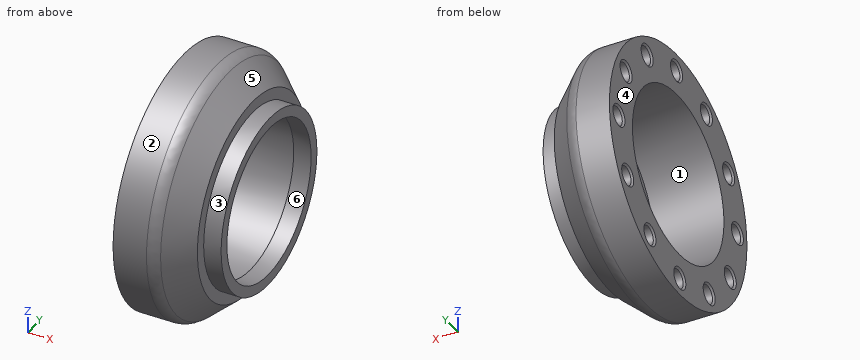
```python
from build123d import *

# Parameters (mm, degrees)
FILLET1_R                    = 10
SKETCH2_R                    = 50.53
SKETCH2_R_2                  = 44.45
BOSS_EXTRUDE1_DEPTH          = 10
SKETCH3_R                    = 5.35
CUT_EXTRUDE1_DEPTH           = 19.4
CHAMFER1_SIZE                = 1
CIRPATTERN1_COUNT            = 12
CHAMFER1_OF_CIRPATTERN1_SIZE = 1


with BuildPart() as part:
    # Sketch1 → Revolve1 (revolve)
    with BuildSketch(Plane.XY):
        Polygon((0, 48.25), (40, 48.25), (40, 57.15), (23, 72.5), (0, 72.5), align=None)
    revolve(axis=Axis((0, 0, 0), (1, 0, 0)))

    # Fillet1
    fillet1_edges = [part.edges().sort_by_distance(p)[0] for p in [
        (23, -72.5, 0),
    ]]
    fillet(fillet1_edges, radius=FILLET1_R)

    # Sketch2 → Boss-Extrude1 (add)
    with BuildSketch(Plane(origin=(40, 0, 0), x_dir=(0, 0, -1), z_dir=(1, 0, 0))):
        Circle(SKETCH2_R)
        Circle(SKETCH2_R_2, mode=Mode.SUBTRACT)
    extrude(amount=BOSS_EXTRUDE1_DEPTH)

    # Sketch3 → Cut-Extrude1 (cut)
    with BuildSketch(Plane.ZY):
        with Locations((-1.718407093, 62.47637215)):
            Circle(SKETCH3_R)
    cut_extrude1 = extrude(amount=-CUT_EXTRUDE1_DEPTH, mode=Mode.SUBTRACT)

    # Chamfer1
    chamfer1_edges = [part.edges().sort_by_distance(p)[0] for p in [
        (0, 62.47637215, -7.068407093),
    ]]
    chamfer(chamfer1_edges, length=CHAMFER1_SIZE)

    # CirPattern1: Cut-Extrude1 ×12 about axis
    cirpattern1_axis = Axis((0, 0, 0), (1, 0, 0))
    for i in range(1, CIRPATTERN1_COUNT):
        add(cut_extrude1.rotate(cirpattern1_axis, i * 360 / CIRPATTERN1_COUNT), mode=Mode.SUBTRACT)

    # Chamfer1 of CirPattern1
    chamfer1_of_cirpattern1_edges = [part.edges().sort_by_distance(p)[0] for p in [
        (0, 57.640328965, 25.116765969),
        (0, 37.359606182, 50.571921872),
        (0, 7.068407093, 62.47637215),
        (0, -25.116765969, 57.640328965),
        (0, -50.571921872, 37.359606182),
        (0, -62.47637215, 7.068407093),
        (0, -57.640328965, -25.116765969),
        (0, -37.359606182, -50.571921872),
        (0, -7.068407093, -62.47637215),
        (0, 25.116765969, -57.640328965),
        (0, 50.571921872, -37.359606182),
    ]]
    chamfer(chamfer1_of_cirpattern1_edges, length=CHAMFER1_OF_CIRPATTERN1_SIZE)


solid = part.part
```
The model under review builds one solid part; all positions refer to its coordinate system, in mm. Face numbers are marked on the shaded views. A direction names the side the tool comes from. Coordinates: 2 decimals unless noted, no trailing zeros. Loops run counter-clockwise (first coordinate to the right, second up) from the corner with the lowest first, then second, coordinate; pieces in that order, holes last. Notation, with made-up numbers: (74, 76.25) -> (80, 76.25) arc R17 cw to (80, 100.25) -> close; hole circle Ø6 at (71.5, 45.5). An arc over 180 degrees is marked (long way). Answer as CSV lines item,"result".
Item 1: Take a section at A-A, the plane x = 4. Count the separate pieces of the cut face and the enclosed holes in it, and give its area (3 significant figures).
Results below:
separate pieces,"1"
enclosed holes,"13"
area,"8,120 mm2"
Item 2: Insertion check: pin 1 (3 mm diameter, centred on y = -54.5, z = 33.5, fed in from -X); pin 2 (12 mm diameter, centred on y = 54, z = 23, fed in from +X); pin 3 (9.5 mm diameter, centred on y = 1.72, z = 62.48, fed in from +X). Each pin has a flat end and moves straight along its axis. Give the tip position at first contact, or say it passes through.
Results below:
pin 1,"stops at x = 19.4"
pin 2,"stops at x = 40"
pin 3,"stops at x = 39.33"
Item 3: Take a section at C-C, the plane x = 36. State the section outline as (y, z) points, and give its area (3 significant figures).
Results below:
outline,"circle Ø121.52 at (0, 0); hole circle Ø96.5 at (0, 0)"
area,"4,280 mm2"
Item 4: Machinability: for the marked faces 1, 2 and 3, which of the approach directions +Z, -Z, +X, -X, +Y, -Y give a long, thin tool a straight path to every point of the face, cutting with its end or side? Answer none if there is none.
Results below:
face 1,"-X"
face 2,"+X, -X"
face 3,"+X"
Item 5: Take a section at B-B, the plane x = 47.5. State the section outline as (y, z) points, and give its area (3 significant figures).
Results below:
outline,"circle Ø101.06 at (0, 0); hole circle Ø88.9 at (0, 0)"
area,"1,810 mm2"
Item 6: For L1, parallel to Y at x = 19, z = 6; L2, parallel to X at y = -50, z = 26; L3, parallel to Y at x = 38.5, z = -9, list the stretches that pass through material, from the lowest coordinate up.
Results below:
L1,"y = -72.25 to -65.68, -59.27 to -47.88, 47.88 to 72.25"
L2,"x = 0 to 40"
L3,"y = -57.81 to -47.4, 47.4 to 57.81"
Item 7: Draft analysis for pull direction Z (two halves, no side actions). For the marked faces 4, 5 and 6, state which applies: +Z half, -Z half, draft (parallel to the pull), parting line (faces both ways), or undercut.
Results below:
face 4,"draft"
face 5,"parting line"
face 6,"undercut"
